Design review of the part built by this model. Coordinates are the model's own, in mm. Face numbers are marked on the shaded views. A direction names the side the tool comes from. Round coordinates to 2 decimals unless told otherwise and drop trailing zeros. Order: outer loops, then holes, each group sorted by start corner. A loop starts at its lowest first (then second) coordinate and runs counter-clockwise, first axis right, second up.
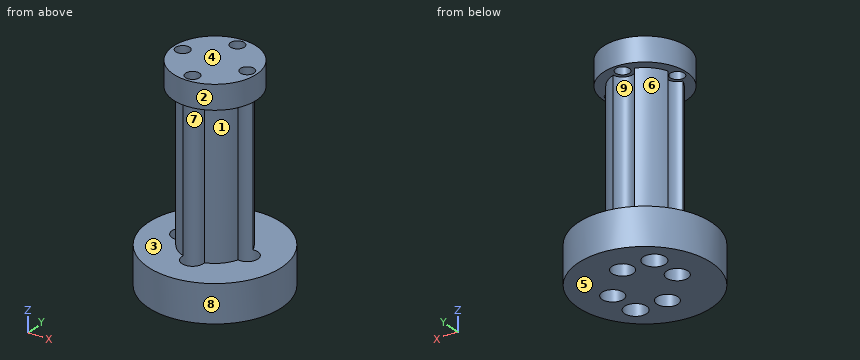
from build123d import *

# Parameters (mm, degrees)
SKETCH1_R           = 12.5
BOSS_EXTRUDE1_DEPTH = 7
SKETCH2_R           = 6
BOSS_EXTRUDE2_DEPTH = 27.5
SKETCH3_R           = 2
CUT_EXTRUDE1_DEPTH  = 35.5
SKETCH4_R           = 2.07
CUT_EXTRUDE2_DEPTH  = 5
SKETCH5_R           = 7.8
BOSS_EXTRUDE3_DEPTH = 4.5
SKETCH6_R           = 1.3
CUT_EXTRUDE3_DEPTH  = 4.5


with BuildPart() as part:
    # Sketch1 → Boss-Extrude1 (new body)
    with BuildSketch(Plane.XY):
        Circle(SKETCH1_R)
    extrude(amount=BOSS_EXTRUDE1_DEPTH)

    # Sketch2 → Boss-Extrude2 (add)
    with BuildSketch(Plane.XY.offset(7)):
        Circle(SKETCH2_R)
    extrude(amount=BOSS_EXTRUDE2_DEPTH)

    # Sketch3 → Cut-Extrude1 (cut, through all)
    with BuildSketch(Plane.XY.offset(34.5)):
        with Locations((0, 6)):
            Circle(SKETCH3_R)
        with Locations((6, 0)):
            Circle(SKETCH3_R)
        with Locations((0, -6)):
            Circle(SKETCH3_R)
        with Locations((-6, 0)):
            Circle(SKETCH3_R)
    extrude(amount=-CUT_EXTRUDE1_DEPTH, mode=Mode.SUBTRACT)

    # Sketch4 → Cut-Extrude2 (cut)
    with BuildSketch(Plane(origin=(0, 0, 0), x_dir=(-1, 0, 0), z_dir=(0, 0, -1))):
        with Locations((5.727564928, 5.727564928)):
            Circle(SKETCH4_R)
        with Locations((-5.727564928, -5.727564928)):
            Circle(SKETCH4_R)
    extrude(amount=-CUT_EXTRUDE2_DEPTH, mode=Mode.SUBTRACT)

    # Sketch5 → Boss-Extrude3 (add)
    with BuildSketch(Plane.XY.offset(34.5)):
        Circle(SKETCH5_R)
    extrude(amount=BOSS_EXTRUDE3_DEPTH)

    # Sketch6 → Cut-Extrude3 (cut)
    with BuildSketch(Plane.XY.offset(39)):
        with Locations((-6, 0)):
            Circle(SKETCH6_R)
        with Locations((0, 6)):
            Circle(SKETCH6_R)
        with Locations((6, 0)):
            Circle(SKETCH6_R)
        with Locations((0, -6)):
            Circle(SKETCH6_R)
    extrude(amount=-CUT_EXTRUDE3_DEPTH, mode=Mode.SUBTRACT)


solid = part.part
1) Clearance check with flat-ended pins moving along their axes: P1, Ø1, axis at y = 4, z = 28, coming from the -X side; P2, Ø8, axis at x = -4, z = 29.5, coming from the -Y side; P3, Ø1.5, axis at y = -2.5, z = 11.5, coming from the -X side. State where each tip first meets the part, or that it passes through.
Results:
P1: stops at x = -4.87
P2: stops at y = -5.67
P3: stops at x = -5.67
2) For the marked faces 1, 2, 3, 4 and 5, list the 3-axis set-ups (+Z, -Z, +X, -X, +Y, -Y) from which the entire face can be reached by the end or side of a thin tool; tool diameter is ignored.
Results:
face 1: +X, -Y
face 2: +Z
face 3: none
face 4: +Z, +X, -X, +Y, -Y
face 5: -Z, +X, -X, +Y, -Y
3) Take a section at D-D on y = -9.5. Give the boundary of the cut face in (x, z), plus the area to 3 significant figures.
Results:
outline: (-8.12, 0) - (8.12, 0) - (8.12, 7) - (-8.12, 7) - close
area: 114 mm2
4) Take a section at A-A on y = 0. Give the boundary of the cut face in (x, z).
Results:
outline: (-12.5, 0) - (-8, 0) - (-8, 7) - (-12.5, 7) - close; (-7.8, 34.5) - (-7.3, 34.5) - (-7.3, 39) - (-7.8, 39) - close; (-4.7, 34.5) - (-4, 34.5) - (-4, 0) - (4, 0) - (4, 34.5) - (4.7, 34.5) - (4.7, 39) - (-4.7, 39) - close; (7.3, 34.5) - (7.8, 34.5) - (7.8, 39) - (7.3, 39) - close; (8, 0) - (12.5, 0) - (12.5, 7) - (8, 7) - close
5) The part is to be moulded in two halves that separate along Y. For the marked faces 6, 7, 8 and 9, say which applies: released by +Y, released by -Y, zero draft, split by the parting line, or undercut.
Results:
face 6: released by +Y
face 7: undercut
face 8: split by the parting line
face 9: undercut
6) Take a section at C-C on z = 23.5. Give the boundary of the cut face in (x, y).
Results:
outline: (-5.67, -1.97) arc R6 ccw to (-1.97, -5.67) arc R2 cw to (1.97, -5.67) arc R6 ccw to (5.67, -1.97) arc R2 cw to (5.67, 1.97) arc R6 ccw to (1.97, 5.67) arc R2 cw to (-1.97, 5.67) arc R6 ccw to (-5.67, 1.97) arc R2 cw to start
7) To check wall thickness, follow line 1 along Z through (x, y) = (5.25, -3); line 2 along Z through (x, y) = (-6.5, -8.75); line 3 along X through (y, z) = (0, 22.5). State the ranges of each line that lie inside material, in increasing order.
Results:
line 1: z = 0 to 7, 34.5 to 39
line 2: z = 0 to 7
line 3: x = -4 to 4
